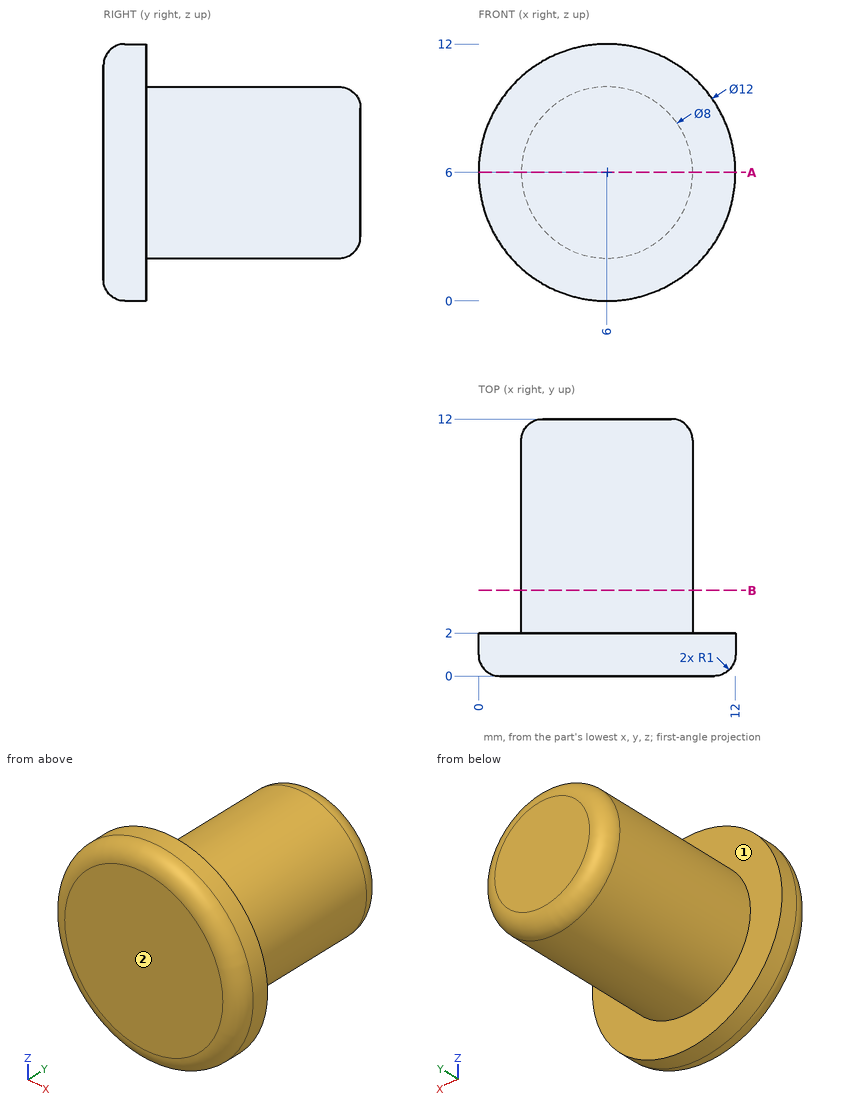
Part print with two shaded views. Sizes in mm from the minimum x, y, z corner. A direction names the side the tool comes from. Round coordinates to 2 decimals unless told otherwise and drop trailing zeros. Loops run counter-clockwise (first coordinate to the right, second up) from the corner with the lowest first, then second, coordinate; pieces in that order, holes last. Notation, with made-up numbers: (9.25, 23) - (38.25, 23) arc R18 cw to (38.25, 31) - close; hole circle Ø1 at (6, 2.25). An arc over 180 degrees is marked (long way). Answer as a JSON object with one key per item and string values.
Item 1: Wall check: L1, parallel to Y at x = 5, z = 10; L2, parallel to Z at x = 7.5, y = 6.25; L3, parallel to Z at x = 5, y = 6.5. Give the ranges that are in metal, low to high.
Output:
{"L1": "0 to 2", "L2": "2.29 to 9.71", "L3": "2.13 to 9.87"}
Item 2: Band-saw the part on A-A on z = 6. List the corners of the cut face in (x, y), plus the area to 3 significant figures.
Output:
{"outline": "(0, 1) arc R1 ccw to (1, 0) - (11, 0) arc R1 ccw to (12, 1) - (12, 2) - (10, 2) - (10, 11) arc R1 ccw to (9, 12) - (3, 12) arc R1 ccw to (2, 11) - (2, 2) - (0, 2) - close", "area": "103 mm2"}
Item 3: Tool access for the marked faces 1 and 2: list every direction of +Z, -Z, +X, -X, +Y, -Y with a clear straight run to the whole face (end or side of a thin tool).
Output:
{"face 1": "+Y", "face 2": "+Z, -Z, +X, -X, -Y"}
Item 4: Band-saw the part on B-B on y = 4. List the corners of the cut face in (x, z), plus the area to 3 significant figures.
Output:
{"outline": "circle Ø8 at (6, 6)", "area": "50.3 mm2"}
Item 5: Pin check, flat tips, straight feed: pin 1 (3 mm diameter, centred on y = 2, z = 8.5, fed in from -X); pin 2 (2 mm diameter, centred on y = 6.5, z = 5, fed in from -X). Stop position of each tip, or through.
Output:
{"pin 1": "x = 0.08", "pin 2": "x = 2"}
